Verification items for the finished model (mm, model axes). A direction names the side the tool comes from. Give positions to 0.01 mm unless a question says otherwise; leave off trailing zeros. Write each loop counter-clockwise with the first axis right and the second up, starting at its lowest first coordinate (ties: lowest second). Pieces come first, ordered by that corner, then holes.
from build123d import *

# Parameters (mm, degrees)
SKETCH1_W           = 14
SKETCH1_H           = 25
BOSS_EXTRUDE1_DEPTH = 3
SKETCH3_W           = 3
SKETCH3_H           = 3
SKETCH3_H_2         = 4
CUT_EXTRUDE2_DEPTH  = 3
SKETCH4_W           = 3
SKETCH4_H           = 4
BOSS_EXTRUDE2_DEPTH = 3


with BuildPart() as part:
    # Sketch1 → Boss-Extrude1 (new body)
    with BuildSketch(Plane.XY):
        Rectangle(SKETCH1_W, SKETCH1_H)
    extrude(amount=BOSS_EXTRUDE1_DEPTH)

    # Sketch3 → Cut-Extrude2 (cut)
    with BuildSketch(Plane.XY.offset(3)):
        with Locations((-5.5, 11)):
            Rectangle(SKETCH3_W, SKETCH3_H)
        with Locations((-5.5, 4)):
            Rectangle(SKETCH3_W, SKETCH3_H)
        with Locations((-5.5, -3)):
            Rectangle(SKETCH3_W, SKETCH3_H)
        with Locations((-5.5, -10.5)):
            Rectangle(SKETCH3_W, SKETCH3_H_2)
    extrude(amount=-CUT_EXTRUDE2_DEPTH, mode=Mode.SUBTRACT)

    # Sketch4 → Boss-Extrude2 (add)
    with BuildSketch(Plane.XY.offset(3)):
        with Locations((8.5, 7.5)):
            Rectangle(SKETCH4_W, SKETCH4_H)
        with Locations((8.5, 0.5)):
            Rectangle(SKETCH4_W, SKETCH4_H)
        with Locations((8.5, -6.5)):
            Rectangle(SKETCH4_W, SKETCH4_H)
    extrude(amount=-BOSS_EXTRUDE2_DEPTH)


solid = part.part
Item 1: Set-up check for faces 5 (the face through (-4, 11, 2)), 6 (the face through (-6, -8.5, 2)), 7 (the face through (-4, -3, 2)): record each of +Z, -Z, +X, -X, +Y, -Y from which the full face is reachable in a straight line by a thin tool's end or side.
Answer key:
face 5: +Z, -Z, -X, +Y
face 6: +Z, -Z, -X, -Y
face 7: +Z, -Z, -X
Item 2: Release check for a two-part mould opening along Y. For faces 1 (the face through (7, -3, 1)), 2 (the face through (8, 5.5, 2)), 3 (the face through (-7, 7, 1)), 4 (the face through (8, 9.5, 2)) record: released by +Y, released by -Y, zero draft, split by the parting line, or undercut.
Answer key:
face 1: undercut
face 2: undercut
face 3: zero draft
face 4: released by +Y
Item 3: Depth check by flat-ended pin: pin 1 (1.5 mm diameter, centred on x = -5, z = 2, fed in from +Y); pin 2 (0.9 mm diameter, centred on y = -2.5, z = 1, fed in from +X); pin 3 (1.5 mm diameter, centred on y = -3, z = 2, fed in from -X). Enter the tip coordinate at first touch or a pass-through.
Answer key:
pin 1: stops at y = 9.5
pin 2: stops at x = 7
pin 3: stops at x = -4
Item 4: Scan lines: line 1 along Y through (x, z) = (7.25, 2.25); line 2 along X through (y, z) = (11, 2.5). Record each from-to range of solid material in increasing order.
Answer key:
line 1: y = -8.5 to -4.5, -1.5 to 2.5, 5.5 to 9.5
line 2: x = -4 to 7
Item 5: Sectioned sample at A-A on x = -5.5. Record the cut outline in (y, z).
Answer key:
outline: (-8.5, 0) - (-4.5, 0) - (-4.5, 3) - (-8.5, 3) - close; (-1.5, 0) - (2.5, 0) - (2.5, 3) - (-1.5, 3) - close; (5.5, 0) - (9.5, 0) - (9.5, 3) - (5.5, 3) - close
Item 6: Sectioned sample at C-C on y = 4.25. Record the cut outline in (x, z), then the cut area to 3 significant figures.
Answer key:
outline: (-4, 0) - (7, 0) - (7, 3) - (-4, 3) - close
area: 33.0 mm2
Item 7: Sectioned sample at B-B on z = 0.95. Record the cut outline in (x, y).
Answer key:
outline: (-7, -8.5) - (-4, -8.5) - (-4, -12.5) - (7, -12.5) - (7, -8.5) - (10, -8.5) - (10, -4.5) - (7, -4.5) - (7, -1.5) - (10, -1.5) - (10, 2.5) - (7, 2.5) - (7, 5.5) - (10, 5.5) - (10, 9.5) - (7, 9.5) - (7, 12.5) - (-4, 12.5) - (-4, 9.5) - (-7, 9.5) - (-7, 5.5) - (-4, 5.5) - (-4, 2.5) - (-7, 2.5) - (-7, -1.5) - (-4, -1.5) - (-4, -4.5) - (-7, -4.5) - close
